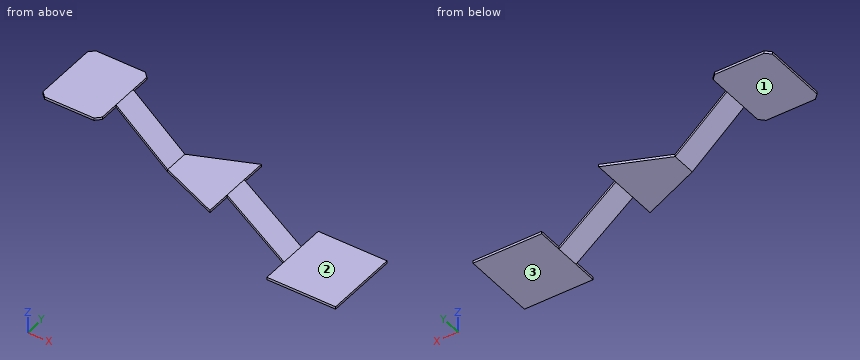
from build123d import *

# Parameters (mm, degrees)
F2_W      = 127
F2_H      = 12.7
F4_W      = 127
F4_H      = 12.7
F7_FACE_W = 127
F7_FACE_H = 12.7
F6_W      = 381
F6_H      = 12.7
F9_W      = 381
F9_H      = 12.7
F10_DEPTH = 304.8
F11_SIZE  = 25.4
F13_W     = 127
F13_H     = 12.7
F15_W     = 381
F15_H     = 12.7
F16_DEPTH = 353.06


with BuildPart() as f7:
    # F2 (on line) → F7 section 0
    with BuildSketch(Plane(origin=(-457.2, 0, 0), x_dir=(0, -1, 0), z_dir=(-1, 0, 0))):
        with Locations((0, 228.6)):
            Rectangle(F2_W, F2_H)
    # F4 (on line) → F7 section 1
    with BuildSketch(Plane(origin=(-191.3811564445, 0, 0), x_dir=(0, -1, 0), z_dir=(-1, 0, 0))):
        Rectangle(F4_W, F4_H)
    loft()

    # F7_face (on face) → F8 section 0
    with BuildSketch(Plane.YZ.offset(-191.3811564445)):
        Rectangle(F7_FACE_W, F7_FACE_H)
    # F6 (on line) → F8 section 1
    with BuildSketch(Plane(origin=(113.4188435555, 0, 0), x_dir=(0, -1, 0), z_dir=(-1, 0, 0))):
        Rectangle(F6_W, F6_H)
    loft()

    # F9 (on line) → F10 (join, through all)
    with BuildSketch(Plane(origin=(-457.2, 0, 0), x_dir=(0, -1, 0), z_dir=(-1, 0, 0))):
        with Locations((0, 228.6)):
            Rectangle(F9_W, F9_H)
    extrude(amount=F10_DEPTH)

    # F11
    f11_edges = [f7.edges().sort_by_distance(p)[0] for p in [
        (-457.2, -190.5, 228.6),
        (-762, -190.5, 228.6),
        (-457.2, 190.5, 228.6),
        (-762, 190.5, 228.6),
    ]]
    chamfer(f11_edges, length=F11_SIZE)

    # F14: sweep along a path in F0
    with BuildLine(Plane.XZ) as f14_path:
        Line((113.4188435555, 0), (406.4, -228.6))
    # F13 (on line) → F14 (sweep)
    with BuildSketch(Plane.YZ.offset(406.4)):
        with Locations((0, -228.6)):
            Rectangle(F13_W, F13_H)
    sweep(path=f14_path.line)

    # F15 (on line) → F16 (join)
    with BuildSketch(Plane.YZ.offset(406.4)):
        with Locations((0, -228.6)):
            Rectangle(F15_W, F15_H)
    extrude(amount=F16_DEPTH)


solid = f7.part
Design review of the part built by this model. Coordinates are the model's own, in mm. Face numbers are marked on the shaded views. A direction names the side the tool comes from. Coordinates: 2 decimals unless noted, no trailing zeros. Loops run counter-clockwise (first coordinate to the right, second up) from the corner with the lowest first, then second, coordinate; pieces in that order, holes last. Notation, with made-up numbers: (-29, 52.5) - (-15, 52.5) arc R7 ccw to (-15, 59.5) - close; hole circle Ø1 at (-16.75, 89). An arc over 180 degrees is marked (long way). Use CSV: the item, a comma, the result in double quotes. Start each with the question number.
1. To check wall thickness, follow probe 1 along Z at (x, y) = (453, 132); probe 2 along Z at (x, y) = (20, 67.5); probe 3 along X at (y, z) = (-153.5, -6). State the ranges of each line that lie inside material, in increasing order.
2. Add section B-B on z = -118.5. Give the boundary of the cut face in (x, y), plus the area to 3 significant figures.
3. Add section A-A on y = 146. Count the separate pieces of the cut face and the enclosed holes in it, plus the area to 3 significant figures.
4. Clearance check with flat-ended pins moving along their axes: pin 1 (4 mm diameter, centred on y = -123, z = -231.5, fed in from -X); pin 2 (8 mm diameter, centred on x = -24, y = -113.5, fed in from +Z); pin 3 (14 mm diameter, centred on y = -118, z = -2.5, fed in from +X). State where each tip first meets the part, or that it passes through.
5. For the marked faces 1, 2 and 3, list the 3-axis set-ups (+Z, -Z, +X, -X, +Y, -Y) from which the entire face can be reached by the end or side of a thin tool; tool diameter is ignored.
Resolved:
1,probe 1,"-234.95 to -222.25"
1,probe 2,"-6.35 to 6.35"
1,probe 3,"24.62 to 113.42"
2,outline,"(257.15, -63.5) - (273.43, -63.5) - (273.43, 63.5) - (257.15, 63.5) - close"
2,area,"2,070 mm2"
3,separate pieces,"3"
3,enclosed holes,"0"
3,area,"9,710 mm2"
4,pin 1,"x = 406.4"
4,pin 2,"z = 6.35"
4,pin 3,"x = 113.42"
5,face 1,"-Z, -X, +Y, -Y"
5,face 2,"+Z, +X, +Y, -Y"
5,face 3,"-Z, +X, -X, +Y, -Y"
